Geometry check sheet. Reference: the model listing, model coordinates, mm. A direction names the side the tool comes from. Round coordinates to 2 decimals unless told otherwise and drop trailing zeros. Write each loop counter-clockwise with the first axis right and the second up, starting at its lowest first coordinate (ties: lowest second). Pieces come first, ordered by that corner, then holes. Notation, with made-up numbers: M -8,21.25 L 27,21.25 A23 ccw 27,58.25 Z; hole C 44.25,33.25 d2. An arc over 180 degrees is marked long. One line per item, written item: value. Start each with the question number.
1. Scan lines: probe 1 along X at (y, z) = (1.8, -17); probe 2 along Z at (x, y) = (8, 3); probe 3 along Z at (x, y) = (11.75, 5.5). Record each from-to range of solid material in increasing order. Write a range as [from, to].
2. Release check for a two-part mould opening along Z. For faces 1 (the flat face through (8, 12, -34)), 2 (the flat face through (10, 0, -21)), 3 (the conical face through (8.1, 8.1, -17.7)) record: pulls with the +Z half, pulls with the -Z half, needs draft (parallel to the pull), parting line crosses it, or undercut.
3. Section check C-C (z = -6.5). Record the boundary of the cut face in (x, y).
4. Section check B-B (x = 13). Record the boundary of the cut face in (y, z), and give its area (3 significant figures).
5. Access from +Z, -Z, +X, -X, +Y, -Y to the whole of each face (thin tool, end or side, straight path). Record for faces 4 (the flat face through (8, 12, 0)), 5 (the cylindrical face through (7.453, 3.042, -21.164)).
6. Section check A-A (y = 3.5). Record the boundary of the cut face in (x, z), and give its area (3 significant figures).
from build123d import *

# Parameters (mm, degrees)
SKETCH1_W                = 16
SKETCH1_H                = 34
BOSS_EXTRUDE1_DEPTH      = 25
BOSS_EXTRUDE2_DEPTH      = 16
M8_CLEARANCE_HOLE1_D     = 8.4
M8_CLEARANCE_HOLE1_DEPTH = 6
M8_CLEARANCE_HOLE1_TIP   = 2.5236146


with BuildPart() as part:
    # Sketch1 → Boss-Extrude1 (new body)
    with BuildSketch(Plane(origin=(0, 0, 0), x_dir=(1, 0, 0), z_dir=(0, 1, 0))):
        with Locations((8, 17)):
            Rectangle(SKETCH1_W, SKETCH1_H)
    extrude(amount=BOSS_EXTRUDE1_DEPTH)

    # Sketch2 → Boss-Extrude2 (add)
    with BuildSketch(Plane(origin=(16, 0, 0), x_dir=(0, 0, -1), z_dir=(1, 0, 0))):
        with BuildLine():
            Line((0, 25), (34, 25))
            ThreePointArc((34, 25), (17, 29.405882918), (0, 25))
        make_face()
    extrude(amount=-BOSS_EXTRUDE2_DEPTH)

    # M8 Clearance Hole1
    with Locations(Plane(origin=(0, 0, 0), x_dir=(-1, 0, 0), z_dir=(0, -1, 0))):
        with Locations((-8, 17)):
            Hole(M8_CLEARANCE_HOLE1_D / 2, depth=M8_CLEARANCE_HOLE1_DEPTH)
            with Locations((0, 0, -(M8_CLEARANCE_HOLE1_DEPTH + M8_CLEARANCE_HOLE1_TIP / 2))):  # 118° drill point
                Cone(0, M8_CLEARANCE_HOLE1_D / 2, M8_CLEARANCE_HOLE1_TIP, mode=Mode.SUBTRACT)


solid = part.part
Result sheet:
1. probe 1: x = [0, 3.8], [12.2, 16]
1. probe 2: z = [-34, -21.2], [-12.8, 0]
1. probe 3: z = [-34, -18.89], [-15.11, 0]
2. face 1: pulls with the -Z half
2. face 2: needs draft
2. face 3: undercut
3. outline: M 0,0 L 16,0 L 16,27.79 L 0,27.79 Z
4. outline: M 0,-34 L 25,-34 A35 ccw 25,0 L 0,0 Z
4. area: 951 mm2
5. face 4: +Z, +X, -X, +Y, -Y
5. face 5: -Y
6. outline: M 0,-34 L 16,-34 L 16,0 L 0,0 Z; hole C 8,-17 d8.4
6. area: 489 mm2
